Read the model definition and answer for the solid it produces. Units are mm, in the model's axes. A direction names the side the tool comes from. Coordinates: 2 decimals unless noted, no trailing zeros. Order: outer loops, then holes, each group sorted by start corner. A loop starts at its lowest first (then second) coordinate and runs counter-clockwise, first axis right, second up.
from build123d import *

# Parameters (mm, degrees)
SKETCH_1_R               = 11.5
SKETCH_1_R_2             = 6.5
EXTRUDE_1_DEPTH          = 8
SKETCH_2_R               = 1.5
CUT_EXTRUDE_2_DEPTH      = 3
PATTERN_CIRCULAR_1_COUNT = 4


with BuildPart() as part:
    # 草图1 → 拉伸1 (new body)
    with BuildSketch(Plane(origin=(0, 0, 0), x_dir=(0, 0, -1), z_dir=(1, 0, 0))):
        Circle(SKETCH_1_R)
        Circle(SKETCH_1_R_2, mode=Mode.SUBTRACT)
    extrude(amount=EXTRUDE_1_DEPTH)

    # 草图2 → 拉伸2 (cut)
    with BuildSketch(Plane(origin=(8, 0, 0), x_dir=(0, 0, -1), z_dir=(1, 0, 0))):
        with Locations((0, 9)):
            Circle(SKETCH_2_R)
    cut_extrude_2 = extrude(amount=-CUT_EXTRUDE_2_DEPTH, mode=Mode.SUBTRACT)

    # 阵列(圆周)1: 拉伸2 ×4 about axis
    pattern_circular_1_axis = Axis((0, 0, 0), (1, 0, 0))
    for i in range(1, PATTERN_CIRCULAR_1_COUNT):
        add(cut_extrude_2.rotate(pattern_circular_1_axis, i * 360 / PATTERN_CIRCULAR_1_COUNT), mode=Mode.SUBTRACT)


solid = part.part
Q1. The part is cut by section C-C, the plane x = 6. Determine the outline of the cut face in (y, z).
Q2. Each of these flat-tipped pins is pushed along its axis until it touches: P1, Ø4, axis at x = 4.5, z = -6.5, coming from the -Y side; P2, Ø4, axis at x = 3.5, z = -4, coming from the +Y side; P3, Ø1.5, axis at y = -9, z = -0.5, coming from the +X side. Where does it stop, or does it pass through?
Q3. The part is cut by section B-B, the plane z = 0.25. Determine the outline of the cut face in (x, y).
Q4. Which of the six approach directions +Z, -Z, +X, -X, +Y, -Y give full straight-line access (tool end or side, diameter ignored) to faces 1 (the flat face through (5, -9, 0)), 2 (the flat face through (0, -5, -5))?
Q5. The part is cut by section D-D, the plane z = 9. Determine the outline of the cut face in (x, y).
Q6. Determine the mould class of faces 3 (the flat face through (8, -5, -5)), 4 (the cylindrical face through (3.9, 11.4, 1.5)), 5 (the cylindrical face through (3.944, -3.955, 5.158)) for opening direction Y: +Y half, -Y half, draft (parallel to the pull), parting line (faces both ways), or undercut.
Q7. Straight lines are drawn through the part: L1, parallel to Y at x = 0.5, z = -5.25; L2, parallel to Z at x = 7.25, y = -5.75; L3, parallel to Y at x = 3.5, z = -2.25. For each, find the intervals that lie inside material, in ascending order.
Q8. The part is cut by section A-A, the plane y = 0. Determine the outline of the cut face in (x, z).
Computed values:
1. outline: circle Ø23 at (0, 0); hole circle Ø3 at (-9, 0); hole circle Ø13 at (0, 0); hole circle Ø3 at (0, -9); hole circle Ø3 at (0, 9); hole circle Ø3 at (9, 0)
2. P1: stops at y = -10.58
2. P2: stops at y = 11.32
2. P3: stops at x = 5
3. outline: (0, -11.5) - (8, -11.5) - (8, -10.48) - (5, -10.48) - (5, -7.52) - (8, -7.52) - (8, -6.5) - (0, -6.5) - close; (0, 6.5) - (8, 6.5) - (8, 7.52) - (5, 7.52) - (5, 10.48) - (8, 10.48) - (8, 11.5) - (0, 11.5) - close
4. face 1: +X
4. face 2: +Z, -Z, -X, +Y, -Y
5. outline: (0, -7.16) - (8, -7.16) - (8, -1.5) - (5, -1.5) - (5, 1.5) - (8, 1.5) - (8, 7.16) - (0, 7.16) - close
6. face 3: draft
6. face 4: parting line
6. face 5: undercut
7. L1: y = -10.23 to -3.83, 3.83 to 10.23
7. L2: z = -9.96 to -3.03, 3.03 to 9.96
7. L3: y = -11.28 to -6.1, 6.1 to 11.28
8. outline: (0, -11.5) - (8, -11.5) - (8, -10.5) - (5, -10.5) - (5, -7.5) - (8, -7.5) - (8, -6.5) - (0, -6.5) - close; (0, 6.5) - (8, 6.5) - (8, 7.5) - (5, 7.5) - (5, 10.5) - (8, 10.5) - (8, 11.5) - (0, 11.5) - close
